The model under review builds one solid part; all positions refer to its coordinate system, in mm. A direction names the side the tool comes from. Coordinates: 2 decimals unless noted, no trailing zeros. Loops run counter-clockwise (first coordinate to the right, second up) from the corner with the lowest first, then second, coordinate; pieces in that order, holes last. Notation, with made-up numbers: M 24.25,87.5 L 69.25,87.5 A18 cw 69.25,96.5 Z; hole C -0.5,60 d3. An arc over 180 degrees is marked long. Write item = value, one per line. Start each with the question number.
Q1. We need section A-A on z = -21. Give the boundary of the cut face in (x, y) (3 decimals).
Q2. We need section C-C on z = 39.5. Give the boundary of the cut face in (x, y).
Q3. For faces 4 (the face through (60.125, 6, 19)), 5 (the face through (-1, 6, 52)), list the 3-axis set-ups (+Z, -Z, +X, -X, +Y, -Y) from which the entire face can be reached by the end or side of a thin tool; tool diameter is ignored.
Q4. Wall thickness on probe 1 along X at (y, z) = (6.5, 39.5); probe 2 along Z at (x, y) = (67.5, 7); probe 3 along X at (y, z) = (4.75, 22.5) (3 decimals): over which ranges is each line inside the solid? List them lowest first.
Q5. We need section B-B on x = -67.5. Give the boundary of the cut face in (y, z), and give its area (3 significant figures).
Q6. We need section D-D on y = 2. Count the separate pieces of the cut face and the enclosed holes in it, and give its area (3 significant figures).
Q7. Clearance check with a flat-ended pin moving along its axis: pin 1 Ø4 at (x, z) = (-67.5, -39.5) entering from +Y (3 decimals). State where the tip first meets the part, or that it passes through.
Q8. Mouldability with a two-part tool opening along X and no side actions: class faces 1 (the face through (-80, 6, -1)), 2 (the face through (48.94, 6.08, 5.04)), 3 (the face through (80, 6, 1)) as released by +X, released by -X, zero draft, split by the parting line, or undercut.
Autodesk Inventor part; units mm, degrees
ref_plane "YZ Plane" through (0, 0, 0) normal (1, 0, 0) x (0, 1, 0)
ref_plane "XZ Plane" through (0, 0, 0) normal (0, 1, 0) x (-1, 0, 0)
ref_plane "XY Plane" through (0, 0, 0) normal (0, 0, 1) x (1, 0, 0)
sketch "Sketch1" plane through (0, 0, 0) normal (0, 1, 0) x (-1, 0, 0)
  line L0 (80, 52) -> (-80, 52)
  line L1 (-80, 52) -> (-80, -52)
  line L2 (-80, -52) -> (80, -52)
  line L3 (80, -52) -> (80, 52)
  line L4 (80, 52) -> (-80, -52) construction
  line L5 (-80, 52) -> (80, -52) construction
  point P0 (0, 0)
  dimension "d0" = 160
  dimension "d1" = 104
extrude "Extrusion1" add sketch "Sketch1" along normal blind 12
sketch "Sketch2" plane through (0, 12, 0) normal (0, 1, 0) x (1, 0, 0)
  line L0 (-80, 52) -> (-80, -52)
  line L1 (80, 52) -> (-80, 52)
  line L2 (-38.125, 26.75) -> (-38.125, 11)
  line L3 (-60.875, 11) -> (-60.875, 26.75)
  arc A0 (-38.125, 26.75) -> (-60.875, 26.75) centre (-49.5, 18.875) ccw
  arc A1 (-60.875, 11) -> (-38.125, 11) centre (-49.5, 18.875) ccw
  point P0 (0, 0)
  dimension "d39" = 22.75
  dimension "d40" = 15.75
  dimension "d41" = 19.125
  dimension "d42" = 7.875
  dimension "d43" = 33.125
extrude "Extrusion2" cut sketch "Sketch2" against normal up to next
pattern_linear "Rectangular Pattern1" count 4 spacing -32.75 along (-1, 0, 0) count 2 spacing 37.75 along (0, 0, 1) of "Extrusion2"
sketch "Sketch4" plane through (0, 12, 0) normal (0, 1, 0) x (1, 0, 0)
  line L0 (-80, 52) -> (-80, -52)
  line L1 (80, 52) -> (-80, 52)
  line L2 (80, -52) -> (80, 52)
  line L3 (-80, -52) -> (80, -52)
  point P0 (0, 0)
  point P1 (-67.5, 39.5)
  point P2 (67.5, 39.5)
  point P3 (67.5, -39.5)
  point P4 (-67.5, -39.5)
  dimension "d24" = 12.5
  dimension "d25" = 12.5
  dimension "d26" = 12.5
  dimension "d27" = 12.5
  dimension "d28" = 12.5
  dimension "d29" = 12.5
  dimension "d30" = 12.5
  dimension "d31" = 12.5
hole "Hole1" at (-67.5, 12, -39.5) at (67.5, 12, -39.5) at (67.5, 12, 39.5) at (-67.5, 12, 39.5) direction (0, -1, 0) diameter 6.756 depth 25.4
fillet "Fillet1" radius 2 4 edges at (-80, 6, 52) (80, 6, 52) (80, 6, -52) (-80, 6, -52)
properties part number "4_OM_VialPlate_0.25mmReduce"
Returned:
q1.outline = M -80,0 L -60.875,0 L -60.875,12 L -80,12 Z; M -38.125,0 L -28.125,0 L -28.125,12 L -38.125,12 Z; M -5.375,0 L 4.625,0 L 4.625,12 L -5.375,12 Z; M 27.375,0 L 37.375,0 L 37.375,12 L 27.375,12 Z; M 60.125,0 L 80,0 L 80,12 L 60.125,12 Z
q2.outline = M -80,0 L -70.88,0 L -70.88,12 L -80,12 Z; M -64.12,0 L 64.12,0 L 64.12,12 L -64.12,12 Z; M 70.88,0 L 80,0 L 80,12 L 70.88,12 Z
q3.face_4 = +Y, -Y
q3.face_5 = +Z, +X, -X, +Y, -Y
q4.probe_1 = -80 to -70.88, -64.12 to 64.12, 70.88 to 80
q4.probe_2 = -52 to -42.88, -36.12 to 36.12, 42.88 to 52
q4.probe_3 = -80 to -60.875, -38.125 to -28.125, -5.375 to 4.625, 27.375 to 37.375, 60.125 to 80
q5.outline = M 0,-52 L 12,-52 L 12,-42.88 L 0,-42.88 Z; M 0,-36.12 L 12,-36.12 L 12,36.12 L 0,36.12 Z; M 0,42.88 L 12,42.88 L 12,52 L 0,52 Z
q5.area = 1,090 mm^2
q6.separate_pieces = 1
q6.enclosed_holes = 12
q6.area = 12,100 mm^2
q7.pin_1 = through
q8.face_1 = released by -X
q8.face_2 = undercut
q8.face_3 = released by +X
